from build123d import *

# Parameters (mm, degrees)
RESSALTO_EXTRUS_O1_DEPTH                            = 98
ESBO_O4_W                                           = 33
ESBO_O4_H                                           = 22
CORTE_EXTRUS_O3_DEPTH                               = 25
ESBO_O10_W                                          = 12
ESBO_O10_H                                          = 4
CORTE_EXTRUS_O8_DEPTH                               = 122.545423608
ESBO_O11_R                                          = 1.6
CORTE_EXTRUS_O9_DEPTH                               = 20
ESBO_O12_W                                          = 22
ESBO_O12_H                                          = 40
CORTE_EXTRUS_O10_DEPTH                              = 10
FILETE1_R                                           = 2.5
ESCAREADO_PARA_PARAFUSO_ALLEN_SEXTAVADO_D           = 4.3
ESCAREADO_PARA_PARAFUSO_ALLEN_SEXTAVADO_CSINK_D     = 8.96
ESCAREADO_PARA_PARAFUSO_ALLEN_SEXTAVADO_CSINK_ANGLE = 90
ESBO_O15_W                                          = 4
ESBO_O15_H                                          = 22
CORTE_EXTRUS_O11_DEPTH                              = 137.386546257
ESBO_O16_W                                          = 59.5
ESBO_O16_H                                          = 54
ESBO_O16_R                                          = 2.15
CORTE_EXTRUS_O12_DEPTH                              = 137.386546257
CHANFRO1_SIZE                                       = 10
CHANFRO1_SIZE2                                      = 7.180150431
CORTE_EXTRUS_O14_DEPTH                              = 102.622518505
CORTE_EXTRUS_O14_DEPTH_BACK                         = 102.622518505
CHANFRO2_SIZE                                       = 8
CHANFRO2_SIZE_2                                     = 9.267647445
CORTE_EXTRUS_O15_REACH                              = 121.956
ESBO_O19_R                                          = 1.5


with BuildPart() as part:
    # Esboço1 → Ressalto-extrusão1 (new body)
    with BuildSketch(Plane.XY):
        Polygon((0, 0), (94, 0), (75.862520314, 12.7), (0, 12.7), align=None)
    extrude(amount=RESSALTO_EXTRUS_O1_DEPTH)

    # Esboço4 → Corte-extrusão3 (cut)
    with BuildSketch(Plane(origin=(0, 12.7, 0), x_dir=(1, 0, 0), z_dir=(0, 1, 0))):
        with Locations((16.5, -87)):
            Rectangle(ESBO_O4_W, ESBO_O4_H)
        with Locations((16.5, -11)):
            Rectangle(ESBO_O4_W, ESBO_O4_H)
        with Locations((53.5, -87)):
            Rectangle(ESBO_O4_W, ESBO_O4_H)
        with Locations((53.5, -11)):
            Rectangle(ESBO_O4_W, ESBO_O4_H)
    extrude(amount=-CORTE_EXTRUS_O3_DEPTH, mode=Mode.SUBTRACT)

    # Esboço10 → Corte-extrusão8 (cut, through all)
    with BuildSketch(Plane.XY.offset(76)):
        with Locations((16.5, 10.7)):
            Rectangle(ESBO_O10_W, ESBO_O10_H)
        with Locations((53.5, 10.7)):
            Rectangle(ESBO_O10_W, ESBO_O10_H)
    extrude(amount=-CORTE_EXTRUS_O8_DEPTH, mode=Mode.SUBTRACT)

    # Esboço11 → Corte-extrusão9 (cut)
    with BuildSketch(Plane(origin=(0, 12.7, 0), x_dir=(1, 0, 0), z_dir=(0, 1, 0))):
        with Locations(Location((29.25, -26.5, 0), (0, 0, 180))):
            Circle(ESBO_O11_R)
        with Locations(Location((29.25, -71.5, 0), (0, 0, 180))):
            Circle(ESBO_O11_R)
        with Locations(Location((3.75, -71.5, 0), (0, 0, 180))):
            Circle(ESBO_O11_R)
        with Locations(Location((3.75, -26.5, 0), (0, 0, 180))):
            Circle(ESBO_O11_R)
        with Locations(Location((40.75, -26.5, 0), (0, 0, 180))):
            Circle(ESBO_O11_R)
        with Locations(Location((66.25, -26.5, 0), (0, 0, 180))):
            Circle(ESBO_O11_R)
        with Locations(Location((66.25, -71.5, 0), (0, 0, 180))):
            Circle(ESBO_O11_R)
        with Locations(Location((40.75, -71.5, 0), (0, 0, 180))):
            Circle(ESBO_O11_R)
    extrude(amount=-CORTE_EXTRUS_O9_DEPTH, mode=Mode.SUBTRACT)

    # Esboço12 → Corte-extrusão10 (cut)
    with BuildSketch(Plane(origin=(0, 12.7, 0), x_dir=(1, 0, 0), z_dir=(0, 1, 0))):
        with Locations((35, -49)):
            Rectangle(ESBO_O12_W, ESBO_O12_H)
    extrude(amount=-CORTE_EXTRUS_O10_DEPTH, mode=Mode.SUBTRACT)

    # Filete1
    filete1_edges = [part.edges().sort_by_distance(p)[0] for p in [
        (46, 7.7, 29),
        (46, 7.7, 69),
        (24, 7.7, 69),
        (24, 7.7, 29),
    ]]
    fillet(filete1_edges, radius=FILETE1_R)

    # Escareado para parafuso Allen sextavado escareado de M41 (through all)
    with Locations(Plane(origin=(0, 0, 0), x_dir=(-1, 0, 0), z_dir=(0, -1, 0))):
        with Locations((-66.25, -71.5), (-66.25, -26.5), (-40.75, -26.5), (-29.25, -26.5), (-29.25, -71.5), (-40.75, -71.5), (-3.75, -71.5), (-3.75, -26.5)):
            CounterSinkHole(ESCAREADO_PARA_PARAFUSO_ALLEN_SEXTAVADO_D / 2, ESCAREADO_PARA_PARAFUSO_ALLEN_SEXTAVADO_CSINK_D / 2, counter_sink_angle=ESCAREADO_PARA_PARAFUSO_ALLEN_SEXTAVADO_CSINK_ANGLE)

    # Esboço15 → Corte-extrusão11 (cut, through all)
    with BuildSketch(Plane(origin=(0, 12.7, 0), x_dir=(1, 0, 0), z_dir=(0, 1, 0))):
        with Locations((35, -11)):
            Rectangle(ESBO_O15_W, ESBO_O15_H)
        with Locations((35, -87)):
            Rectangle(ESBO_O15_W, ESBO_O15_H)
    extrude(amount=-CORTE_EXTRUS_O11_DEPTH, mode=Mode.SUBTRACT)

    # Esboço16 → Corte-extrusão12 (cut, through all)
    # profile 1 of 2: a face of its own
    with BuildSketch(Plane(origin=(0, 12.7, 0), x_dir=(1, 0, 0), z_dir=(0, 1, 0))):
        with Locations((29.75, -49)):
            Rectangle(ESBO_O16_W, ESBO_O16_H)
    # profile 2 of 2: a face of its own
    with BuildSketch(Plane(origin=(0, 12.7, 0), x_dir=(1, 0, 0), z_dir=(0, 1, 0))):
        Polygon((70, -42), (70, -22), (59.5, -22), (59.5, -76), (70, -76), (70, -56), (65, -56), (65, -42), align=None)
        with Locations((66.25, -71.5)):
            Circle(ESBO_O16_R, mode=Mode.SUBTRACT)
        with Locations((66.25, -26.5)):
            Circle(ESBO_O16_R, mode=Mode.SUBTRACT)
    extrude(amount=-CORTE_EXTRUS_O12_DEPTH, mode=Mode.SUBTRACT)

    # Chanfro1
    chanfro1_edges = [part.edges().sort_by_distance(p)[0] for p in [
        (94, 0, 49),
    ]]
    chanfro1_side = [part.faces().sort_by_distance(p)[0] for p in [
        (81.603595513, 0, 49),
    ]]
    chamfer(chanfro1_edges, length=CHANFRO1_SIZE, length2=CHANFRO1_SIZE2, reference=chanfro1_side[0])

    # Esboço18 → Corte-extrusão14 (cut, two sides: drawn at the far end of the back side and taken through both)
    with BuildSketch(Plane.XY.offset(49).offset(-CORTE_EXTRUS_O14_DEPTH_BACK)):
        Polygon((73.318031781, 10.208958991), (85.605312446, 1.605312446), (84.16928236, 0.16928236), (72.170878909, 8.570654902), align=None)
    extrude(amount=CORTE_EXTRUS_O14_DEPTH + CORTE_EXTRUS_O14_DEPTH_BACK, mode=Mode.SUBTRACT)

    # Chanfro2
    # the kernel refuses this chamfer: 9.267647445, 8 mm, written as the material it takes off along each edge
    with BuildSketch(Plane(origin=(88.118365096, 4.118365096, -23.833451274), x_dir=(-0.6804962674600086, -0.7327515472334374, 0), z_dir=(0, 0, 1))) as chanfro2_piece_1_section:
        Polygon((CHANFRO2_SIZE * 0.999317113267, -CHANFRO2_SIZE * 0.0369500626806), (CHANFRO2_SIZE_2 * 0.137140887434, -CHANFRO2_SIZE_2 * 0.990551551958), (0, 0), align=None)
    chanfro2_piece_1 = extrude(amount=145.666902548, mode=Mode.PRIVATE)
    chanfro2_piece_1 = split(chanfro2_piece_1, bisect_by=Plane(origin=(81.702068422, 1.896844157, 49), z_dir=(0.5735764363510464, 0.8191520442889916, 0)), keep=Keep.TOP, mode=Mode.PRIVATE)
    add(chanfro2_piece_1, mode=Mode.SUBTRACT)

    # Esboço19 → Corte-extrusão15 (cut, up to next)
    with BuildSketch(Plane(origin=(30.925053264, 44.165553177, 0), x_dir=(0.819152044288991, -0.5735764363510472, 0), z_dir=(0.5735764363510472, 0.819152044288991, 0)), mode=Mode.PRIVATE) as corte_extrus_o15_sk1:
        with Locations(Location((57.358517859, -74, 0), (0, 0, 180))):
            Circle(ESBO_O19_R)
    corte_extrus_o15_tool1 = extrude(corte_extrus_o15_sk1.sketch, amount=-CORTE_EXTRUS_O15_REACH, mode=Mode.PRIVATE) & part.part
    # Esboço19 → Corte-extrusão15 (cut, up to next)
    with BuildSketch(Plane(origin=(30.925053264, 44.165553177, 0), x_dir=(0.819152044288991, -0.5735764363510472, 0), z_dir=(0.5735764363510472, 0.819152044288991, 0)), mode=Mode.PRIVATE) as corte_extrus_o15_sk2:
        with Locations(Location((57.358517859, -49, 0), (0, 0, 180))):
            Circle(ESBO_O19_R)
    corte_extrus_o15_tool2 = extrude(corte_extrus_o15_sk2.sketch, amount=-CORTE_EXTRUS_O15_REACH, mode=Mode.PRIVATE) & part.part
    # Esboço19 → Corte-extrusão15 (cut, up to next)
    with BuildSketch(Plane(origin=(30.925053264, 44.165553177, 0), x_dir=(0.819152044288991, -0.5735764363510472, 0), z_dir=(0.5735764363510472, 0.819152044288991, 0)), mode=Mode.PRIVATE) as corte_extrus_o15_sk3:
        with Locations(Location((57.358517859, -24, 0), (0, 0, 180))):
            Circle(ESBO_O19_R)
    corte_extrus_o15_tool3 = extrude(corte_extrus_o15_sk3.sketch, amount=-CORTE_EXTRUS_O15_REACH, mode=Mode.PRIVATE) & part.part
    add(corte_extrus_o15_tool1.solids().sort_by_distance((77.9104, 11.266059, 74))[0], mode=Mode.SUBTRACT)
    add(corte_extrus_o15_tool2.solids().sort_by_distance((77.9104, 11.266059, 49))[0], mode=Mode.SUBTRACT)
    add(corte_extrus_o15_tool3.solids().sort_by_distance((77.9104, 11.266059, 24))[0], mode=Mode.SUBTRACT)


solid = part.part
Here's how the part is built. I have some questions about the finished solid (model axes, mm). A direction names the side the tool comes from. Round coordinates to 2 decimals unless told otherwise and drop trailing zeros. Write each loop counter-clockwise with the first axis right and the second up, starting at its lowest first coordinate (ties: lowest second). Pieces come first, ordered by that corner, then holes.
1. Will these pins go through, and if not, where does the flat tip stop? pin 1 Ø4 at (y, z) = (4.5, 31.5) entering from -X; pin 2 Ø1.5 at (x, y) = (69, 11) entering from -Z; pin 3 Ø5.5 at (x, y) = (67, 8) entering from +Z.
2. For faces 5 (the flat face through (73, 12.7, 48)), 6 (the flat face through (67, 6, 42)), 7 (the flat face through (78.254, 4.311, 48.314)), 8 (the flat face through (70, 6, 77)), which set-ups out of +Z, -Z, +X, -X, +Y, -Y let a thin tool reach every point of the face, with its end or its side?
3. Suppose I cut it at D-D (z = 53). List the corners of the cut face in (x, y) for me.
4. I need wall thicknesses on L1, parallel to Y at x = 72.5, z = 4.5; L2, parallel to Y at x = 73.25, z = 28.5; L3, parallel to Z at x = 69.5, y = 3. Which ranges of each line are inside material? Lowest first, please.
5. If we mould it in two halves opening along Z, with no side actions, what happens to faces 1 (the cylindrical face through (76.26, 10.315, 75.265)), 2 (the flat face through (77.3, 7.42, 48.31)), 3 (the flat face through (68, 6, 56)), 4 (the cylindrical face through (76.26, 10.315, 25.265))? For each: released by +Z, released by -Z, zero draft, split by the parting line, or undercut.
6. Suppose I cut it at A-A (y = 6.25). List the corners of the cut face in (x, z) for me, and give its area (3 significant figures).
7. Suppose I cut it at C-C (x = 67.25). List the corners of the cut face in (y, z) for me.
8. Suppose I cut it at B-B (z = 37.5). List the corners of the cut face in (x, y) for me.
Answer sheet:
1. pin 1: stops at x = 70
1. pin 2: stops at z = 42
1. pin 3: stops at z = 56
2. face 5: +Z, -Z, +X, -X, +Y
2. face 6: -Z, -X, +Y, -Y
2. face 7: +Z, -Z
2. face 8: +Z, -X, +Y, -Y
3. outline: (65, 0) - (84, 0) - (84.17, 0.17) - (72.17, 8.57) - (73.32, 10.21) - (81.39, 4.56) - (80.53, 9.43) - (75.86, 12.7) - (65, 12.7) - close
4. L1: y = 0 to 8.34, 9.04 to 12.7
4. L2: y = 0 to 7.82, 10.11 to 12.7
4. L3: z = 42 to 56
5. face 1: undercut
5. face 2: zero draft
5. face 3: released by +Z
5. face 4: undercut
6. outline: (65, 42) - (70, 42) - (70, 0) - (75.49, 0) - (75.49, 98) - (70, 98) - (70, 56) - (65, 56) - close; (78.97, 0) - (81.09, 0) - (81.09, 98) - (78.97, 98) - close
6. area: 815 mm2
7. outline: (0, 42) - (12.7, 42) - (12.7, 56) - (0, 56) - close
8. outline: (70, 0) - (84, 0) - (84.17, 0.17) - (72.17, 8.57) - (73.32, 10.21) - (81.39, 4.56) - (80.53, 9.43) - (75.86, 12.7) - (70, 12.7) - close
